CAD build for the part. Positions are in the model's coordinates, mm. Face numbers are marked on the shaded views. A direction names the side the tool comes from. Round coordinates to 2 decimals unless told otherwise and drop trailing zeros. Loops run counter-clockwise (first coordinate to the right, second up) from the corner with the lowest first, then second, coordinate; pieces in that order, holes last. Notation, with made-up numbers: M 10,-32.75 L 37,-32.75 A21 cw 37,-12.75 Z; hole C 34,16.5 d10. An arc over 180 degrees is marked long. Put each result on its own line as item: value. Start each with the question number.
from build123d import *

# Parameters (mm, degrees)
BOSS_EXTRUDE1_DEPTH = 30
BOSS_EXTRUDE3_DEPTH = 10
SKETCH17_R          = 1.655
CUT_EXTRUDE10_DEPTH = 30
CUT_EXTRUDE11_DEPTH = 6
CUT_EXTRUDE12_DEPTH = 1.8
CUT_EXTRUDE13_DEPTH = 7.2
SKETCH24_R          = 7.75
CUT_EXTRUDE15_DEPTH = 19


with BuildPart() as part:
    # Sketch1 → Boss-Extrude1 (new body)
    with BuildSketch(Plane.XY):
        with BuildLine():
            Line((-5.05, 9.05), (5.05, 9.05))
            ThreePointArc((5.05, 9.05), (7.878427125, 7.878427125), (9.05, 5.05))
            Line((9.05, 5.05), (9.05, -5.05))
            ThreePointArc((9.05, -5.05), (7.878427125, -7.878427125), (5.05, -9.05))
            Line((5.05, -9.05), (-5.05, -9.05))
            ThreePointArc((-5.05, -9.05), (-7.878427125, -7.878427125), (-9.05, -5.05))
            Line((-9.05, -5.05), (-9.05, 5.05))
            ThreePointArc((-9.05, 5.05), (-7.878427125, 7.878427125), (-5.05, 9.05))
        make_face()
    extrude(amount=BOSS_EXTRUDE1_DEPTH)

    # Sketch15 → Boss-Extrude3 (add)
    with BuildSketch(Plane.XY):
        with BuildLine():
            Line((-5.05, -9.05), (5.05, -9.05))
            ThreePointArc((5.05, -9.05), (7.878427125, -7.878427125), (9.05, -5.05))
            Line((9.05, -5.05), (9.05, 8))
            ThreePointArc((9.05, 8), (7.878427125, 10.828427125), (5.05, 12))
            Line((5.05, 12), (-5.05, 12))
            ThreePointArc((-5.05, 12), (-7.878427125, 10.828427125), (-9.05, 8))
            Line((-9.05, 8), (-9.05, -5.05))
            ThreePointArc((-9.05, -5.05), (-7.878427125, -7.878427125), (-5.05, -9.05))
        make_face()
    extrude(amount=BOSS_EXTRUDE3_DEPTH)

    # Sketch17 → Cut-Extrude10 (cut)
    with BuildSketch(Plane(origin=(9.05, 0, 0), x_dir=(0, 0, -1), z_dir=(1, 0, 0))):
        with Locations((-3.6, 6.1)):
            Circle(SKETCH17_R)
    extrude(amount=-CUT_EXTRUDE10_DEPTH, mode=Mode.SUBTRACT)

    # Sketch18 → Cut-Extrude11 (cut)
    with BuildSketch(Plane.XY):
        Polygon((-4.996539756, -4.259182236), (-3.851088562, -6.946129507), (-2.048481088, -4.559068161), (-0.563070773, -7.21717083), (0.983895836, -4.624244345), (2.704822485, -7.21717083), (3.469678774, -4.870091009), (4.674482161, -7.026054964), (4.998172504, -5.668676456), (4.998172504, 5.373520003), (-4.996539756, 5.373520003), align=None)
    extrude(amount=CUT_EXTRUDE11_DEPTH, mode=Mode.SUBTRACT)

    # Sketch20 → Cut-Extrude12 (cut)
    with BuildSketch(Plane(origin=(0, 0, 6), x_dir=(-1, 0, 0), z_dir=(0, 0, -1))):
        Polygon((-7, 0), (-7, 13.473809321), (7, 13.473809321), (7, 0), (7, -7.194424303), (-7, -7.194424303), align=None)
    extrude(amount=-CUT_EXTRUDE12_DEPTH, mode=Mode.SUBTRACT)

    # Sketch21 → Cut-Extrude13 (cut)
    with BuildSketch(Plane.XY):
        Polygon((5, 17.493725323), (-5, 17.493725323), (-5, 0), (-5, -0.5), (5, -0.5), (5, 0), align=None)
    extrude(amount=CUT_EXTRUDE13_DEPTH, mode=Mode.SUBTRACT)

    # Sketch24 → Cut-Extrude15 (cut)
    with BuildSketch(Plane.XY.offset(30)):
        Circle(SKETCH24_R)
    extrude(amount=-CUT_EXTRUDE15_DEPTH, mode=Mode.SUBTRACT)


solid = part.part
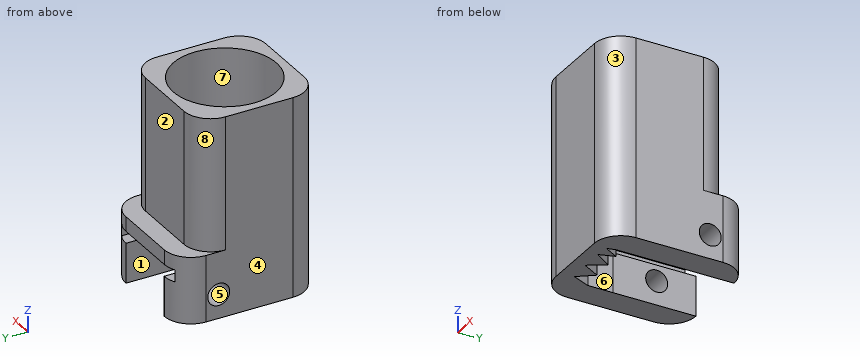
(1) Mould opens along X. For the marked faces 1, 2, 3 and 4 say: +X half, -X half, draft (parallel to the pull), parting line (faces both ways), or undercut.
(2) Cut at D-D on y = -6. List the corners of the cut face in (x, z), and give its area (3 significant figures).
(3) Flat gauge pins, fed straight in: pin 1 Ø2 at (x, z) = (7, 17) entering from -Y; pin 2 Ø0.5 at (x, z) = (-1, 7) entering from +Y; pin 3 Ø3 at (x, y) = (-2.5, -1.5) entering from +Z. Where does each tip first touch, or does it go through?
(4) Cut at A-A on z = 20. List the corners of the cut face in (x, y).
(5) Cut at C-C on x = -5.5. List the corners of the cut face in (y, z) (3 decimals).
(6) Drill centre lines: line 1 along Y through (x, z) = (0, 17); line 2 along Z through (x, y) = (6.25, 10); line 3 along X through (y, z) = (-5.75, 3.5). Where is each one in solid material? Low to high.
(7) Tool access for the marked faces 5, 6, 7 and 8: list every direction of +Z, -Z, +X, -X, +Y, -Y with a clear straight run to the whole face (end or side of a thin tool).
(8) Cut at B-B on y = 6.1. List the corners of the cut face in (x, z) (3 decimals).
Taken from the geometry:
1. face 1: undercut
1. face 2: draft
1. face 3: +X half
1. face 4: -X half
2. outline: M -8.94,0 L -4.25,0 L -4.25,6 L -7,6 L -7,7.8 L 7,7.8 L 7,6 L 4.92,6 L 4.92,0 L 8.94,0 L 8.94,30 L 4.91,30 L 4.91,11 L -4.91,11 L -4.91,30 L -8.94,30 Z; M -3.14,0 L -1.24,0 L -1.24,6 L -3.14,6 Z; M 0.16,0 L 1.9,0 L 1.9,6 L 0.16,6 Z; M 3.1,0 L 4.1,0 L 4.1,6 L 3.1,6 Z
2. area: 297 mm2
3. pin 1: y = -8.94
3. pin 2: y = -7.19
3. pin 3: z = 11
4. outline: M -9.05,-5.05 A4 ccw -5.05,-9.05 L 5.05,-9.05 A4 ccw 9.05,-5.05 L 9.05,5.05 A4 ccw 5.05,9.05 L -5.05,9.05 A4 ccw -9.05,5.05 Z; hole C 0,0 d15.5
5. outline: M -9.025,0 L 11.975,0 L 11.975,6 L -7.194,6 L -7.194,7.8 L 11.975,7.8 L 11.975,10 L 9.025,10 L 9.025,30 L 5.46,30 L 5.46,11 L -5.46,11 L -5.46,30 L -9.025,30 Z; hole C 6.1,3.6 d3.31
6. line 1: -9.05 to -7.75, 7.75 to 9.05
6. line 2: 0 to 6, 7.8 to 10
6. line 3: -8.99 to -4.36, -2.95 to -1.38, 0.31 to 1.73, 3.18 to 3.96, 4.98 to 8.99
7. face 5: +X, -X
7. face 6: -Z, +Y
7. face 7: +Z
7. face 8: +Z, -X, +Y
8. outline: M -9.05,0 L -5,0 L -5,1.945 L -9.05,1.945 Z; M -9.05,5.255 L -5,5.255 L -5,6 L -7,6 L -7,7.8 L 7,7.8 L 7,6 L 5,6 L 5,5.255 L 9.05,5.255 L 9.05,10 L 8.91,10 L 8.91,30 L 4.78,30 L 4.78,11 L -4.78,11 L -4.78,30 L -8.91,30 L -8.91,10 L -9.05,10 Z; M 5,0 L 9.05,0 L 9.05,1.945 L 5,1.945 Z
